from build123d import *

# Parameters (mm, degrees)
BOSS_EXTRUDE1_DEPTH = 18
SKETCH3_R           = 2.5
SKETCH3_R_2         = 3
CUT_EXTRUDE1_DEPTH  = 42.41062241
FILLET1_R           = 3


with BuildPart() as part:
    # Sketch1 → Boss-Extrude1 (new body)
    with BuildSketch(Plane(origin=(0, 0, 0), x_dir=(1, 0, 0), z_dir=(0, 1, 0))):
        Polygon((-8.25, 11.972768964), (-8.25, -27.027231036), (13.25, -11.972768964), (13.25, 11.972768964), (4.25, 11.972768964), (4.25, 30.472768964), (-4.25, 30.472768964), (-4.25, 11.972768964), align=None)
    extrude(amount=BOSS_EXTRUDE1_DEPTH)

    # Sketch3 → Cut-Extrude1 (cut, through all)
    with BuildSketch(Plane.ZY.offset(8.25)):
        with Locations((-21.472768964, 9)):
            Circle(SKETCH3_R)
        with Locations((-1.922768964, 9)):
            Circle(SKETCH3_R_2)
        with Locations((10.077231036, 9)):
            Circle(SKETCH3_R_2)
        with BuildLine():
            Line((-30.472768964, 9), (-30.472768964, 18))
            Line((-30.472768964, 18), (-21.472768964, 18))
            ThreePointArc((-21.472768964, 18), (-27.836729995, 15.363961031), (-30.472768964, 9))
        make_face()
    extrude(amount=-CUT_EXTRUDE1_DEPTH, mode=Mode.SUBTRACT)

    # Fillet1
    fillet1_edges = [part.edges().sort_by_distance(p)[0] for p in [
        (-4.25, 18, -16.722768964),
        (-4.25, 4.5, -30.472768964),
        (-4.25, 15.363961031, -27.836729995),
    ]]
    fillet(fillet1_edges, radius=FILLET1_R)


solid = part.part
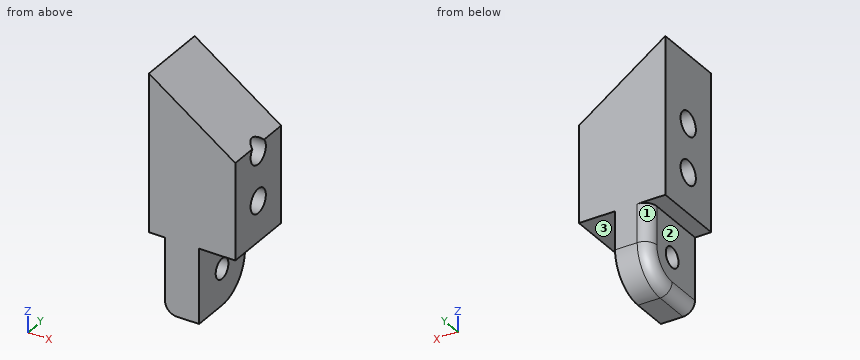
Read the model definition and answer for the solid it produces. Units are mm, in the model's axes. Face numbers are marked on the shaded views. A direction names the side the tool comes from. Give positions to 0.01 mm unless a question says otherwise; leave off trailing zeros. Write each loop counter-clockwise with the first axis right and the second up, starting at its lowest first coordinate (ties: lowest second). Pieces come first, ordered by that corner, then holes. Notation, with made-up numbers: (60, 69) -> (65, 69) arc R15 cw to (65, 91) -> close; hole circle Ø6 at (82.25, 4.5). An arc over 180 degrees is marked (long way). Answer as a JSON object with one key per item and string values. Group by question number.
1) Consider L1, parallel to Z at x = -5.75, y = 9.75; L2, parallel to X at y = 2, z = -15; L3, parallel to Y at x = 0.5, z = -20. Determine where each line is inside the solid, lowest interval first. Write a range as from..to.
2) Find section A-A (y = 1.5). Write down the section's boundary in (x, z), and give its area (3 significant figures).
3) Each of these flat-tipped pins is pushed along its axis until it touches: P1, Ø2, axis at y = 5, z = 18.5, coming from the +X side; P2, Ø3.5, axis at x = -4, y = 9, coming from the -Z side; P3, Ø3, axis at y = 11, z = -19, coming from the +X side; P4, Ø5, axis at y = 9, z = -1.92, coming from the -X side. Where does it stop, or does it pass through?
4) Find section B-B (x = 11). Write down the section's boundary in (y, z).
5) Find section D-D (y = 9.75). Count the separate pieces of the cut face and the enclosed holes in it, and give its area (3 significant figures).
6) A tool of negligible diameter and unlimited length cuts with its end or side. For the marked faces 1, 2 and 3, from which of +Z, -Z, +X, -X, +Y, -Y can it reach the whole face along a straight path? Write none if from no direction.
7) Find section C-C (x = -3.5). Write down the section's boundary in (y, z), and give its area (3 significant figures).
Values follow:
{
 "1": {"L1": "z = -11.97..-4.83, 0.98..7.17, 12.98..25.28", "L2": "x = -4.25..4.25", "L3": "y = 0..6.98, 11.02..18"},
 "2": {"outline": "(-8.25, -11.97) -> (-4.25, -11.97) -> (-4.25, -27.47) arc R3 ccw to (-1.25, -30.47) -> (4.25, -30.47) -> (4.25, -11.97) -> (13.25, -11.97) -> (13.25, 11.97) -> (-8.25, 27.03) -> close", "area": "832 mm2"},
 "3": {"P1": "stops at x = 5.36", "P2": "stops at z = -30.3", "P3": "stops at x = 4.25", "P4": "passes through"},
 "4": {"outline": "(0, -11.97) -> (18, -11.97) -> (18, 13.55) -> (0, 13.55) -> close; hole circle Ø6 at (9, -1.92); hole circle Ø6 at (9, 10.08)"},
 "5": {"separate pieces": "4", "enclosed holes": "0", "area": "542 mm2"},
 "6": {"face 1": "-Z, -X, +Y", "face 2": "-Z, -X, +Y, -Y", "face 3": "-Z, +X, +Y, -Y"},
 "7": {"outline": "(0, -29.46) -> (9, -29.46) arc R7.98 ccw to (16.98, -21.47) -> (16.98, -11.97) -> (18, -11.97) -> (18, 23.7) -> (0, 23.7) -> close; hole circle Ø6 at (9, -1.92); hole circle Ø6 at (9, 10.08); hole circle Ø5 at (9, -21.47)", "area": "849 mm2"}
}
